For this review, take the finished solid that the model builds, in its own axes (mm). Face numbers are marked on the shaded views. A direction names the side the tool comes from. Give positions to 0.01 mm unless a question says otherwise; leave off trailing zeros. Order: outer loops, then holes, each group sorted by start corner. A loop starts at its lowest first (then second) coordinate and runs counter-clockwise, first axis right, second up. Notation, with made-up numbers: (10.5, 89) - (68.5, 89) arc R11 ccw to (68.5, 104) - close; hole circle Ø3 at (49.5, 30.25). An arc over 180 degrees is marked (long way). Use a Markdown table: item, result. Add a question column.
1) Wall thickness on L1, parallel to Y at x = 5, z = 2.3; L2, parallel to Z at x = -1, y = 4: over which ranges is each line inside the solid? List them lowest first.
2) We need section A-A on x = 5.25. Write out the cut boundary in (y, z), then the cut area to 3 significant figures.
3) Machinability: for the marked faces 1, 2 and 3, which of the approach directions +Z, -Z, +X, -X, +Y, -Y give a long, thin tool a straight path to every point of the face, cutting with its end or side? Answer none if there is none.
4) We need section B-B on z = 2.15. Write out the cut boundary in (x, y), then the cut area to 3 significant figures.
```python
from build123d import *

# Parameters (mm, degrees)
PAD001_DEPTH = 1
PAD002_DEPTH = 0.5
FILLET003_R  = 0.2


with BuildPart() as obj1:
    # Sketch008 → Pad001 (new body)
    with BuildSketch(Plane.XY):
        Polygon((-4.5, 5), (5, 0), (-4.5, -5), align=None)
    extrude(amount=PAD001_DEPTH)


with BuildPart() as obj1_1:
    # Body003 placement: moved
    add(obj1.part.moved(Location((0, 0, 2))))


with BuildPart() as obj2:
    # Sketch009 → Pad002 (new body)
    with BuildSketch(Plane.XY.offset(2)):
        Polygon((-5.8, 5.8), (-0.3, 5.8), (-0.3, 0.8), (0.3, 0.8), (0.3, 5.8), (5.8, 5.8), (5.8, 0.3), (0.8, 0.3), (0.8, -0.3), (5.8, -0.3), (5.8, -5.8), (0.3, -5.8), (0.3, -0.8), (-0.3, -0.8), (-0.3, -5.8), (-5.8, -5.8), (-5.8, -0.3), (-0.8, -0.3), (-0.8, 0.3), (-5.8, 0.3), align=None)
    extrude(amount=PAD002_DEPTH)

    # Fusion: union obj1
    add(obj1_1.part)

    # Fillet003
    fillet003_edges = [obj2.edges().sort_by_distance(p)[0] for p in [
        (-3.05, 5.8, 2.5),
        (-5.8, 3.05, 2.5),
        (-0.3, 4.294737, 2.5),
        (-5.15, 0.3, 2.5),
        (5, 0, 2.5),
        (0.25, 2.5, 3),
        (-4.5, 5, 2.75),
        (-4.5, 0, 3),
        (-4.5, -5, 2.75),
        (0.3, 4.136842, 2.5),
        (5.115, 0.3, 2.5),
        (5.8, 3.05, 2.5),
        (3.05, 5.8, 2.5),
        (0.25, -2.5, 3),
        (-5.15, -0.3, 2.5),
        (-5.8, -3.05, 2.5),
        (-3.05, -5.8, 2.5),
        (-0.3, -4.294737, 2.5),
        (5.115, -0.3, 2.5),
        (0.3, -4.136842, 2.5),
        (3.05, -5.8, 2.5),
        (5.8, -3.05, 2.5),
    ]]
    fillet(fillet003_edges, radius=FILLET003_R)


solid = obj2.part
```
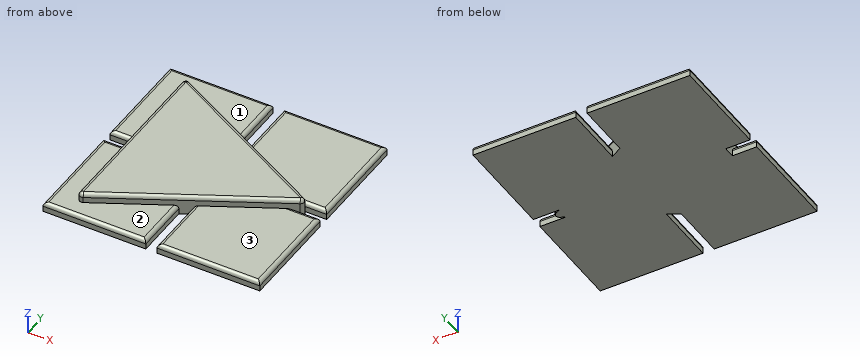
Checked values:
| question | item | result |
|---|---|---|
| 1 | L1 | -5.8 to -0.3, 0.3 to 5.8 |
| 1 | L2 | 2 to 2.5 |
| 2 | outline | (-5.8, 2) - (-0.3, 2) - (-0.3, 2.3) arc R0.2 ccw to (-0.5, 2.5) - (-5.6, 2.5) arc R0.2 ccw to (-5.8, 2.3) - close; (0.3, 2) - (5.8, 2) - (5.8, 2.3) arc R0.2 ccw to (5.6, 2.5) - (0.5, 2.5) arc R0.2 ccw to (0.3, 2.3) - close |
| 2 | area | 5.47 mm² |
| 3 | face 1 | +Z, +Y |
| 3 | face 2 | +Z, -Y |
| 3 | face 3 | +Z, +X, -Y |
| 4 | outline | (-5.8, -5.8) - (-0.3, -5.8) - (-0.3, -2.79) - (0.3, -2.47) - (0.3, -5.8) - (5.8, -5.8) - (5.8, -0.3) - (4.43, -0.3) - (4.66, -0.18) arc R0.2 ccw to (4.66, 0.18) - (4.43, 0.3) - (5.8, 0.3) - (5.8, 5.8) - (0.3, 5.8) - (0.3, 2.47) - (-0.3, 2.79) - (-0.3, 5.8) - (-5.8, 5.8) - (-5.8, 0.3) - (-4.5, 0.3) - (-4.5, -0.3) - (-5.8, -0.3) - close |
| 4 | area | 129 mm² |
